```python
from build123d import *

# Parameters (mm, degrees)
SKETCH_W     = 31.5
SKETCH_H     = 31.5
PAD_DEPTH    = 0.9
SKETCH001_W  = 26
SKETCH001_H  = 26
PAD001_DEPTH = 4
SKETCH002_W  = 25
SKETCH002_H  = 25
PAD002_DEPTH = 4.5
FILLET_R     = 2
FILLET001_R  = 1
CHAMFER_SIZE = 2
FILLET002_R  = 0.5
SKETCH003_R  = 1.18907
POCKET_DEPTH = 2
SKETCH004_R  = 0.5
PAD003_DEPTH = 7


with BuildPart() as part:
    # Sketch → Pad (new body)
    with BuildSketch(Plane.XY):
        with Locations((-15.75, 15.75)):
            Rectangle(SKETCH_W, SKETCH_H)
    extrude(amount=PAD_DEPTH)

    # Sketch001 (on Face5 of Pad) → Pad001 (join)
    with BuildSketch(Plane(origin=(0, 0, 0), x_dir=(1, 0, 0), z_dir=(0, 0, -1))):
        with Locations((-15.75, -15.75)):
            Rectangle(SKETCH001_W, SKETCH001_H)
    extrude(amount=PAD001_DEPTH)

    # Sketch002 (on Face5 of Pad001) → Pad002 (join)
    with BuildSketch(Plane.XY.offset(0.9)):
        with Locations((-15.75, 15.75)):
            Rectangle(SKETCH002_W, SKETCH002_H)
    extrude(amount=PAD002_DEPTH)

    # Fillet
    fillet_edges = [part.edges().sort_by_distance(p)[0] for p in [
        (-3.25, 28.25, 3.15),
        (-3.25, 3.25, 3.15),
        (-28.25, 28.25, 3.15),
        (-28.25, 3.25, 3.15),
    ]]
    fillet(fillet_edges, radius=FILLET_R)

    # Fillet001
    fillet001_edges = [part.edges().sort_by_distance(p)[0] for p in [
        (-15.75, 28.25, 5.4),
        (-27.664214, 27.664214, 5.4),
        (-3.835786, 27.664214, 5.4),
        (-28.25, 15.75, 5.4),
        (-3.25, 15.75, 5.4),
        (-27.664214, 3.835786, 5.4),
        (-3.835786, 3.835786, 5.4),
        (-15.75, 3.25, 5.4),
    ]]
    fillet(fillet001_edges, radius=FILLET001_R)

    # Chamfer
    chamfer_edges = [part.edges().sort_by_distance(p)[0] for p in [
        (-2.75, 2.75, -2),
        (-2.75, 28.75, -2),
        (-28.75, 2.75, -2),
        (-28.75, 28.75, -2),
    ]]
    chamfer(chamfer_edges, length=CHAMFER_SIZE)

    # Fillet002
    fillet002_edges = [part.edges().sort_by_distance(p)[0] for p in [
        (-15.75, 2.75, -4),
        (-27.75, 3.75, -4),
        (-3.75, 3.75, -4),
        (-28.75, 15.75, -4),
        (-2.75, 15.75, -4),
        (-27.75, 27.75, -4),
        (-3.75, 27.75, -4),
        (-15.75, 28.75, -4),
    ]]
    fillet(fillet002_edges, radius=FILLET002_R)

    # Sketch003 (on Face7 of Fillet002) → Pocket (cut)
    with BuildSketch(Plane(origin=(0, 28.75, 0), x_dir=(-1, 0, 0), z_dir=(0, 1, 0))):
        with Locations((15.75, -1.5)):
            Circle(SKETCH003_R)
    extrude(amount=-POCKET_DEPTH, mode=Mode.SUBTRACT)

    # Sketch004 (on Face25 of Pocket) → Pad003 (join)
    with BuildSketch(Plane(origin=(0, 26.75, 0), x_dir=(-1, 0, 0), z_dir=(0, 1, 0))):
        with Locations((15.747266, -1.504022)):
            Circle(SKETCH004_R)
    extrude(amount=PAD003_DEPTH)


solid = part.part
```
Could you check a few things on this model? Use its own coordinates, in mm. A direction names the side the tool comes from. Round coordinates to 2 decimals unless told otherwise and drop trailing zeros. Write each loop counter-clockwise with the first axis right and the second up, starting at its lowest first coordinate (ties: lowest second). Pieces come first, ordered by that corner, then holes. Notation, with made-up numbers: M 39,24 L 56,24 A31 cw 56,63 Z; hole C 2,-4 d10. An arc over 180 degrees is marked long. Answer in a Markdown table with one row per item. Add a question column.
Q1. Will these pins go through, and if not, where does the flat tip stop? pin 1 Ø4 at (x, z) = (-15, -1) entering from -Y; pin 2 Ø0.7 at (x, z) = (-14.5, 0.5) entering from +Y; pin 3 Ø1 at (y, z) = (13, 3.5) entering from +X; pin 4 Ø1 at (y, z) = (11, 2.5) entering from -X.
Q2. On a 3-axis mill with a long thin cutter (end or side, diameter ignored), from which of +Z, -Z, +X, -X, +Y, -Y can I reach the whole of each face in a straight line? I mean faces 4 (the flat face through (-4, 28, -2)), 5 (the flat face through (-15, 26.75, -1)), 6 (the flat face through (-30, 16, 0.9)), 7 (the flat face through (-3.25, 16, 3)), 8 (the cylindrical face through (-3.82, 27.65, 2.67)). Say none if no direction works.
Q3. If we mould it in two halves opening along X, with no side actions, what happens to faces 1 (the flat face through (-31.5, 15.5, 0.4)), 2 (the cylindrical face through (-14.56, 27.76, -1.45)), 3 (the flat face through (-3.7, 3.8, -1.7))? For each: +X half, -X half, draft (parallel to the pull), parting line (faces both ways), or undercut.
Q4. Imagine slicing it at A-A (x = -20). Please give me the cut outline in (y, z), then the cut area to 3 significant figures.
Q5. If I drill on line 1 (Z direction, x = -15.75, y = 27.2); line 2 (Z direction, x = -15.75, y = 28.3); line 3 (Y direction, x = -25, z = -0.75), over which ranges is the centre line in solid material (lowest first)? Write a range as from..to.
Q6. Imagine slicing it at D-D (y = 30). Please give me the cut outline in (x, z), then the cut area to 3 significant figures.
Q7. Imagine slicing it at B-B (y = 15). Please give me the cut outline in (x, z).
Q8. Imagine slicing it at C-C (z = 3). Please give me the cut outline in (x, y), then the cut area to 3 significant figures.
Values:
| question | item | result |
|---|---|---|
| 1 | pin 1 | y = 0 |
| 1 | pin 2 | y = 31.5 |
| 1 | pin 3 | x = -3.25 |
| 1 | pin 4 | x = -28.25 |
| 2 | face 4 | -Z, +X, +Y |
| 2 | face 5 | +Y |
| 2 | face 6 | +Z |
| 2 | face 7 | +Z, +X, +Y, -Y |
| 2 | face 8 | +Z, +X, +Y |
| 3 | face 1 | -X half |
| 3 | face 2 | undercut |
| 3 | face 3 | +X half |
| 4 | outline | M 0,0 L 2.75,0 L 2.75,-3.5 A0.5 ccw 3.25,-4 L 28.25,-4 A0.5 ccw 28.75,-3.5 L 28.75,0 L 31.5,0 L 31.5,0.9 L 28.25,0.9 L 28.25,4.4 A1 ccw 27.25,5.4 L 4.25,5.4 A1 ccw 3.25,4.4 L 3.25,0.9 L 0,0.9 Z |
| 4 | area | 244 mm^2 |
| 5 | line 1 | -4..-2.69, -2..-1, -0.31..5.4 |
| 5 | line 2 | -4..-2.69, -2..-1, -0.31..0.9 |
| 5 | line 3 | 2.75..28.75 |
| 6 | outline | M -31.5,0 L 0,0 L 0,0.9 L -31.5,0.9 Z; C -15.75,-1.5 d1 |
| 6 | area | 29.1 mm^2 |
| 7 | outline | M -31.5,0 L -28.75,0 L -28.75,-3.5 A0.5 ccw -28.25,-4 L -3.25,-4 A0.5 ccw -2.75,-3.5 L -2.75,0 L 0,0 L 0,0.9 L -3.25,0.9 L -3.25,4.4 A1 ccw -4.25,5.4 L -27.25,5.4 A1 ccw -28.25,4.4 L -28.25,0.9 L -31.5,0.9 Z |
| 8 | outline | M -28.25,5.25 A2 ccw -26.25,3.25 L -5.25,3.25 A2 ccw -3.25,5.25 L -3.25,26.25 A2 ccw -5.25,28.25 L -26.25,28.25 A2 ccw -28.25,26.25 Z |
| 8 | area | 622 mm^2 |
